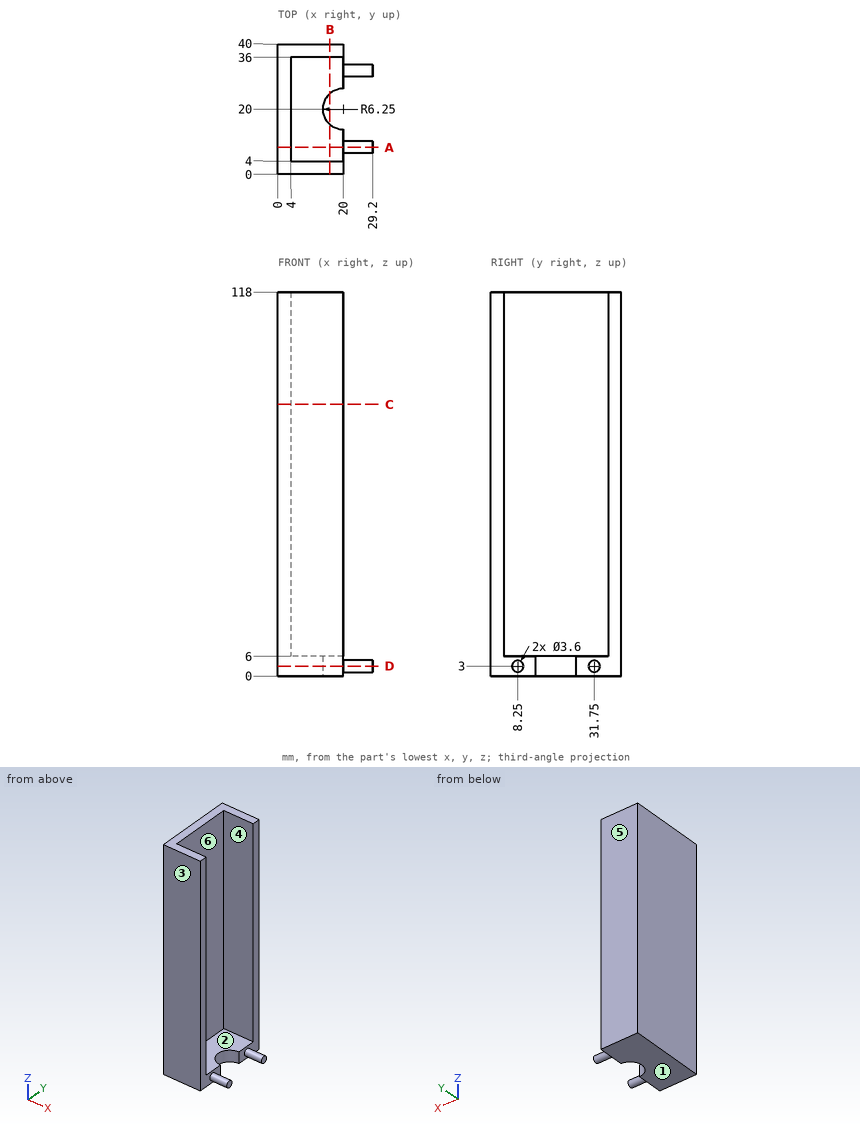
Job drawing, mm, ordinate dimensions from the low corner. One solid piece. A direction names the side the tool comes from. Give positions to 0.01 mm unless a question says otherwise; leave off trailing zeros. Loops run counter-clockwise (first coordinate to the right, second up) from the corner with the lowest first, then second, coordinate; pieces in that order, holes last.
Item 1: Which spindle directions (+Z, -Z, +X, -X, +Y, -Y) get a long thin tool onto all of the face, cutting with end or side? Do the marked faces 5 and 6. Say none if no direction does.
Answers follow:
face 5: +Z, -Z, +X, -X, +Y
face 6: +Z, +X
Item 2: Slice it at A-A, the plane y = 8.25. List the corners of the cut face in (x, z), and give its area (3 significant figures).
Answers follow:
outline: (0, 0) - (20, 0) - (20, 1.2) - (29.2, 1.2) - (29.2, 4.8) - (20, 4.8) - (20, 6) - (4, 6) - (4, 118) - (0, 118) - close
area: 601 mm2
Item 3: Flat gauge pins, fed straight in: pin 1 (8 mm diameter, centred on x = 22, y = 16.5, fed in from +Z); pin 2 (11 mm diameter, centred on y = 36, z = 69.5, fed in from +X); pin 3 (12 mm diameter, centred on x = 21, z = 72.5, fed in from -Y); pin 4 (9.5 mm diameter, centred on y = 17, z = 35, fed in from +X). Where does each tip first touch, or does it go through?
Answers follow:
pin 1: stops at z = 6
pin 2: stops at x = 20
pin 3: stops at y = 0
pin 4: stops at x = 4
Item 4: Pull direction Y, two halves, no side cores. Call the marked faces 1, 2, 3 and 4: released by +Y, released by -Y, zero draft, split by the parting line, or undercut.
Answers follow:
face 1: zero draft
face 2: undercut
face 3: released by -Y
face 4: undercut
Item 5: Drill centre lines: line 1 (Y direction, x = 19.75, z = 13.5); line 2 (X direction, y = 10.5, z = 111.5); line 3 (Z direction, x = 13.25, y = 7.5). Where is each one in solid material? Low to high.
Answers follow:
line 1: y = 0 to 4, 36 to 40
line 2: x = 0 to 4
line 3: z = 0 to 6
Item 6: Slice it at C-C, the plane z = 83.5. List the corners of the cut face in (x, y).
Answers follow:
outline: (0, 0) - (20, 0) - (20, 4) - (4, 4) - (4, 36) - (20, 36) - (20, 40) - (0, 40) - close
Item 7: Slice it at D-D, the plane z = 3. List the corners of the cut face in (x, y).
Answers follow:
outline: (0, 0) - (20, 0) - (20, 6.45) - (29.2, 6.45) - (29.2, 10.05) - (20, 10.05) - (20, 13.75) arc R6.25 cw to (20, 26.25) - (20, 29.95) - (29.2, 29.95) - (29.2, 33.55) - (20, 33.55) - (20, 40) - (0, 40) - close
Item 8: Slice it at B-B, the plane x = 16. List the corners of the cut face in (y, z), and give its area (3 significant figures).
Answers follow:
outline: (0, 0) - (15.2, 0) - (15.2, 6) - (4, 6) - (4, 118) - (0, 118) - close; (24.8, 0) - (40, 0) - (40, 118) - (36, 118) - (36, 6) - (24.8, 6) - close
area: 1,080 mm2
